Could you check a few things on this model? Use its own coordinates, in mm. Face numbers are marked on the shaded views. A direction names the side the tool comes from. Coordinates: 2 decimals unless noted, no trailing zeros. Loops run counter-clockwise (first coordinate to the right, second up) from the corner with the lowest first, then second, coordinate; pieces in that order, holes last. Notation, with made-up numbers: M 73.5,-11.5 L 85.5,-11.5 A14 ccw 85.5,-7.5 Z; hole C 12.25,-10.75 d11. An arc over 180 degrees is marked long. Use one line per item in the form item = value. Start each with the question number.
```python
from build123d import *

# Parameters (mm, degrees)
EXTRUDE_START       = 1
SKETCH_1_W          = 19.9
SKETCH_1_H          = 27.69
EXTRUDE_1_DEPTH     = 7.38
SKETCH_3_R          = 0.75
EXTRUDE_3_DEPTH     = 1
SKETCH_2_R          = 0.25
EXTRUDE_2_DEPTH     = 4
SKETCH_4_R          = 0.75
CUT_EXTRUDE_1_DEPTH = 0.1


with BuildPart() as part:
    # Эскиз1 → Бобышка-Вытянуть1 (new body)
    with BuildSketch(Plane.XY.offset(EXTRUDE_START)):
        Rectangle(SKETCH_1_W, SKETCH_1_H)
    extrude(amount=EXTRUDE_1_DEPTH)

    # Эскиз3 → Бобышка-Вытянуть3 (add)
    with BuildSketch(Plane(origin=(0, 0, 1), x_dir=(-1, 0, 0), z_dir=(0, 0, -1))):
        with Locations((-9.2, 13.095)):
            Circle(SKETCH_3_R)
        with Locations((9.2, 13.095)):
            Circle(SKETCH_3_R)
        with Locations((9.2, -13.095)):
            Circle(SKETCH_3_R)
        with Locations((-9.2, -13.095)):
            Circle(SKETCH_3_R)
    extrude(amount=EXTRUDE_3_DEPTH)

    # Эскиз2 → Бобышка-Вытянуть2 (add)
    with BuildSketch(Plane(origin=(0, 0, 1), x_dir=(-1, 0, 0), z_dir=(0, 0, -1))):
        with Locations((-7.62, -8.89)):
            Circle(SKETCH_2_R)
        with Locations((7.62, -3.81)):
            Circle(SKETCH_2_R)
        with Locations((7.62, -1.27)):
            Circle(SKETCH_2_R)
        with Locations((7.62, 1.27)):
            Circle(SKETCH_2_R)
        with Locations((7.62, 3.81)):
            Circle(SKETCH_2_R)
        with Locations((7.62, 6.35)):
            Circle(SKETCH_2_R)
        with Locations((7.62, 8.89)):
            Circle(SKETCH_2_R)
        with Locations((-7.62, -6.35)):
            Circle(SKETCH_2_R)
        with Locations((-7.62, -3.81)):
            Circle(SKETCH_2_R)
        with Locations((-7.62, -1.27)):
            Circle(SKETCH_2_R)
        with Locations((-7.62, 1.27)):
            Circle(SKETCH_2_R)
        with Locations((-7.62, 3.81)):
            Circle(SKETCH_2_R)
        with Locations((-7.62, 8.89)):
            Circle(SKETCH_2_R)
    extrude(amount=EXTRUDE_2_DEPTH)

    # Эскиз4 → Вырез-Вытянуть1 (cut)
    with BuildSketch(Plane.XY.offset(8.38)):
        with Locations((-7.95, -9.395)):
            Circle(SKETCH_4_R)
        with Locations((7.95, -9.395)):
            Circle(SKETCH_4_R)
        Polygon((-3.10454324, 0.765), (-2.184248514, 1.565), (4.899303826, 1.565), (5.594733216, 0.765), (4.67443849, -0.035), (-2.409113849, -0.035), align=None)
        Polygon((-4.096222413, -9.395), (3.780432652, -9.395), (4.512049983, -8.759014757), (3.674044739, -7.795), (-3.490293806, -7.795), (-4.627637046, -8.783677395), align=None)
        Polygon((5.048482741, -0.37235479), (4.05139953, -7.466970486), (4.889404773, -8.430985243), (5.621022104, -7.795), (6.652963591, -0.45235479), (5.922762731, 0.38764521), align=None)
        Polygon((-4.119895806, 1.933029514), (-3.432572754, 1.14235479), (-2.501550526, 1.951680066), (-1.51139953, 8.996970486), (-2.349404773, 9.960985243), (-3.081022104, 9.325), align=None)
        Polygon((-4.448207492, -0.403029514), (-3.48189803, 0.436970486), (-2.821240109, -0.323029514), (-3.818323321, -7.41764521), (-4.955666561, -8.406322605), (-5.487081194, -7.795), align=None)
        Polygon((-1.240432652, 10.925), (-1.972049983, 10.289014757), (-1.134044739, 9.325), (6.030293806, 9.325), (7.167637046, 10.313677395), (6.636222413, 10.925), align=None)
        Polygon((6.358323321, 8.94764521), (7.495666561, 9.936322605), (8.027081194, 9.325), (6.995139707, 1.98235479), (5.972088006, 1.093029514), (5.354307894, 1.803704239), align=None)
    extrude(amount=-CUT_EXTRUDE_1_DEPTH, mode=Mode.SUBTRACT)


solid = part.part
```
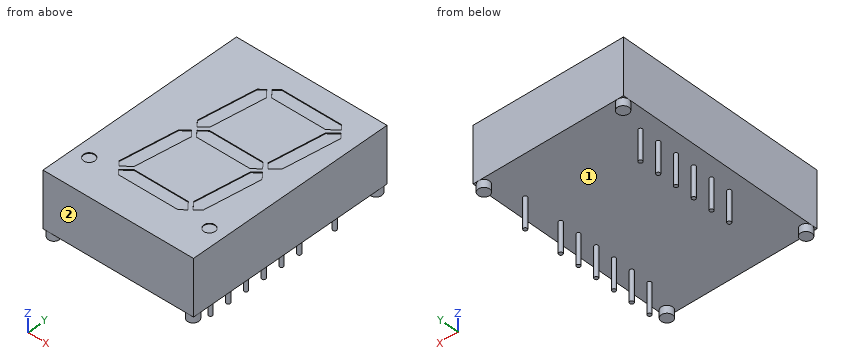
Item 1: Please list where these lines run through material, in increasing order: line 1 along Z through (x, y) = (4.5, 9); line 2 along Z through (x, y) = (-2.5, 5.75).
Item 2: I want a section at A-A (z = -0.5). Count the separate pieces of the cut face and the enclosed holes in it, plus the area to 3 significant figures.
Item 3: I want a section at B-B (y = 8). Write out the boundary of the cut face in (x, z).
Item 4: For the marked faces 1 and 2, which set-ups out of +Z, -Z, +X, -X, +Y, -Y let a thin tool reach every point of the face, with its end or its side?
Item 5: I'm going to push flat-ended pins straight in: P1, Ø0.8, axis at x = 7, y = 7.5, coming from the +Z side; P2, Ø1.6, axis at x = -9.5, y = 13.5, coming from the -Z side; P3, Ø5, axis at x = -1.5, y = 2, coming from the -Z side. Where does each tip first touch, or does it pass through?
Worked answers:
q1.line_1 = 1 to 8.38
q1.line_2 = 1 to 8.28
q2.separate_pieces = 13
q2.enclosed_holes = 0
q2.area = 2.55 mm²
q3.outline = M -9.95,1 L 9.95,1 L 9.95,8.38 L 7.84,8.38 L 7.84,8.28 L 6.23,8.28 L 6.23,8.38 L -1.65,8.38 L -1.65,8.28 L -3.27,8.28 L -3.27,8.38 L -9.95,8.38 Z
q4.face_1 = -Z
q4.face_2 = +Z, -Z, +X, -X, -Y
q5.P1 = 8.28
q5.P2 = 0
q5.P3 = 1
